Check sheet for the modelled part. Datum: model origin and axes. Units: mm. Round coordinates to 2 decimals unless told otherwise and drop trailing zeros. Order: outer loops, then holes, each group sorted by start corner. A loop starts at its lowest first (then second) coordinate and runs counter-clockwise, first axis right, second up. Notation, with made-up numbers: (85, 9) -> (106, 9) arc R14 cw to (106, 20) -> close; hole circle Ø10 at (23, 18). An arc over 180 degrees is marked (long way). Answer in a Markdown table with one row per item.
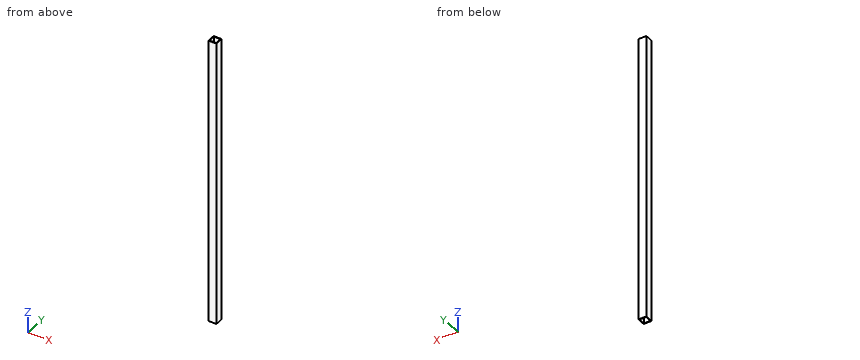
Autodesk Inventor part; units mm, degrees
ref_plane "YZ Plane" through (0, 0, 0) normal (1, 0, 0) x (0, 1, 0)
ref_plane "XZ Plane" through (0, 0, 0) normal (0, 1, 0) x (-1, 0, 0)
ref_plane "XY Plane" through (0, 0, 0) normal (0, 0, 1) x (1, 0, 0)
sketch "Sketch1" plane through (0, 0, 0) normal (0, 0, 1) x (1, 0, 0)
  line L0 (0, 0) -> (50.8, 0)
  line L1 (50.8, 0) -> (50.8, 50.8)
  line L2 (50.8, 50.8) -> (0, 50.8)
  line L3 (0, 50.8) -> (0, 0)
  line L4 (0, 0) -> (4.7625, 0) construction
  line L5 (4.7625, 0) -> (4.7625, 4.7625) construction
  line L6 (4.7625, 4.7625) -> (0, 4.7625) construction
  line L7 (0, 4.7625) -> (0, 0) construction
  line L8 (50.8, 50.8) -> (46.0375, 50.8) construction
  line L9 (46.0375, 50.8) -> (46.0375, 46.0375) construction
  line L10 (46.0375, 46.0375) -> (50.8, 46.0375) construction
  line L11 (50.8, 46.0375) -> (50.8, 50.8) construction
  line L12 (46.0375, 46.0375) -> (4.7625, 46.0375)
  line L13 (4.7625, 46.0375) -> (4.7625, 4.7625)
  line L14 (4.7625, 4.7625) -> (46.0375, 4.7625)
  line L15 (46.0375, 4.7625) -> (46.0375, 46.0375)
  dimension "d0" = 50.8
  dimension "d1" = 50.8
  dimension "d2" = 4.7625
  dimension "d3" = 4.7625
  dimension "d4" = 4.7625
  dimension "d5" = 4.7625
extrude "Extrusion1" add sketch "Sketch1" along normal blind 1828.8
equation "\"d0\" = d1"
equation "\"d2\" = d3"
equation "\"d4\" = d3"
equation "\"d5\" = d3"
properties part number "72in2.0Sq" material "Steel, Mild"
Item 1: Cross-section at C-C (z = 627.5). Record the boundary of the cut face in (x, y).
Result sheet:
| item | result |
|---|---|
| outline | (0, 0) -> (50.8, 0) -> (50.8, 50.8) -> (0, 50.8) -> close; hole (4.76, 4.76) -> (46.04, 4.76) -> (46.04, 46.04) -> (4.76, 46.04) -> close |
Item 2: Scan line: line 1 (Y direction, x = 28, z = 1012.5). Record every from-to range of solid material in increasing order. Write a range as [from, to].
Result sheet:
| item | result |
|---|---|
| line 1 | y = [0, 4.76], [46.04, 50.8] |
Item 3: Cross-section at A-A (y = 15). Record the boundary of the cut face in (x, z), and give its area (3 significant figures).
Result sheet:
| item | result |
|---|---|
| outline | (0, 0) -> (4.76, 0) -> (4.76, 1828.8) -> (0, 1828.8) -> close; (46.04, 0) -> (50.8, 0) -> (50.8, 1828.8) -> (46.04, 1828.8) -> close |
| area | 17,400 mm^2 |
Item 4: Depth check by flat-ended pin: P1, Ø8, axis at x = 40.5, y = 17.5, coming from the -Z side; P2, Ø3, axis at x = 17, z = 1335, coming from the -Y side. Enter the tip coordinate at first touch or a pass-through.
Result sheet:
| item | result |
|---|---|
| P1 | passes through |
| P2 | stops at y = 0 |
